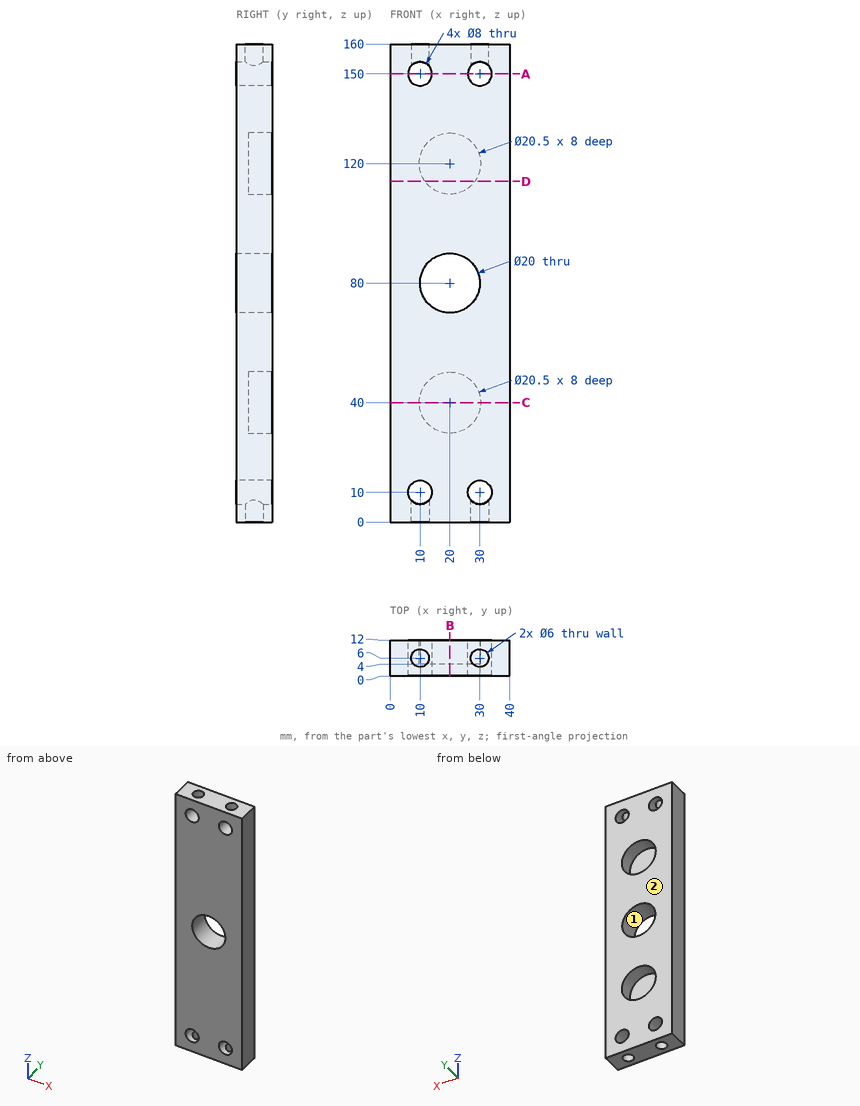
Design review of the part shown in the three views and the two pictorial views. Dimensions are in mm from the part's minimum x, y and z. Give positions to 0.01 mm unless a question says otherwise; leave off trailing zeros. Loops run counter-clockwise (first coordinate to the right, second up) from the corner with the lowest first, then second, coordinate; pieces in that order, holes last. Notation, with made-up numbers: (4.5, 79.5) -> (35.5, 79.5) arc R6 cw to (35.5, 84.5) -> close; hole circle Ø11 at (-38, -3). An arc over 180 degrees is marked (long way). Answer as a JSON object with one key per item and string values. Group by question number.
Q1. Take a section at C-C (z = 40). Write out the cut boundary in (x, y), plus the area to 3 significant figures.
Q2. Take a section at D-D (z = 114). Write out the cut boundary in (x, y).
Q3. Draft analysis for pull direction Z (two halves, no side actions). For the marked faces 1 and 2, state which applies: pulls with the +Z half, pulls with the -Z half, needs draft (parallel to the pull), parting line crosses it, or undercut.
Q4. Insertion check: pin 1 (5 mm diameter, centred on x = 10, y = 6, fed in from -Z); pin 2 (10 mm diameter, centred on x = 24, z = 40, fed in from +Y). Each pin has a flat end and moves straight along its axis. Give the tip position at first contact, or say it passes through.
Q5. Wall thickness on line 1 along X through (y, z) = (5.75, 10); line 2 along Y through (x, z) = (30, 5.25); line 3 along Z through (x, y) = (12, 5.5): over which ranges is each line inside the solid? List them lowest first.
Q6. Take a section at B-B (x = 20). Write out the cut boundary in (y, z).
Q7. Take a section at A-A (z = 150). Write out the cut boundary in (x, y), plus the area to 3 significant figures.
Answer below:
{
 "1": {"outline": "(0, 0) -> (40, 0) -> (40, 12) -> (30.25, 12) -> (30.25, 4) -> (9.75, 4) -> (9.75, 12) -> (0, 12) -> close", "area": "316 mm2"},
 "2": {"outline": "(0, 0) -> (40, 0) -> (40, 12) -> (28.31, 12) -> (28.31, 4) -> (11.69, 4) -> (11.69, 12) -> (0, 12) -> close"},
 "3": {"face 1": "undercut", "face 2": "needs draft"},
 "4": {"pin 1": "stops at z = 13.12", "pin 2": "stops at y = 4"},
 "5": {"line 1": "x = 0 to 6, 14 to 26, 34 to 40", "line 2": "y = 0 to 3, 9 to 12", "line 3": "z = 13.46 to 33.59, 46.41 to 74, 86 to 113.59, 126.41 to 146.54"},
 "6": {"outline": "(0, 0) -> (12, 0) -> (12, 29.75) -> (4, 29.75) -> (4, 50.25) -> (12, 50.25) -> (12, 70) -> (0, 70) -> close; (0, 90) -> (12, 90) -> (12, 109.75) -> (4, 109.75) -> (4, 130.25) -> (12, 130.25) -> (12, 160) -> (0, 160) -> close"},
 "7": {"outline": "(0, 0) -> (6, 0) -> (6, 12) -> (0, 12) -> close; (14, 0) -> (26, 0) -> (26, 12) -> (14, 12) -> close; (34, 0) -> (40, 0) -> (40, 12) -> (34, 12) -> close", "area": "288 mm2"}
}
